from build123d import *

# Parameters (mm, degrees)
BOSS_EXTRUDE1_DEPTH = 3.175
SKETCH3_R           = 6.35
CUT_EXTRUDE2_DEPTH  = 4.175
CUT_EXTRUDE4_DEPTH  = 4.175
SKETCH4_W           = 6.35
SKETCH4_H           = 3.2258
CUT_EXTRUDE3_DEPTH  = 4.175


with BuildPart() as part:
    # Sketch1 → Boss-Extrude1 (new body)
    with BuildSketch(Plane(origin=(0, 0, 0), x_dir=(0, 0, -1), z_dir=(1, 0, 0))):
        with BuildLine():
            Line((20.308664328, 40.617328656), (43.157786531, 40.617328656))
            ThreePointArc((43.157786531, 40.617328656), (60.466141811, 27.624512399), (43.692194932, 13.948725661))
            Line((43.692194932, 13.948725661), (15.586038544, 7.228441393))
            Line((15.586038544, 7.228441393), (15.586038544, -35.582671344))
            Line((15.586038544, -35.582671344), (-17.791335672, -35.582671344))
            Line((-17.791335672, -35.582671344), (-17.791335672, 40.617328656))
            Line((-17.791335672, 40.617328656), (20.308664328, 40.617328656))
        make_face()
    extrude(amount=BOSS_EXTRUDE1_DEPTH)

    # Sketch3 → Cut-Extrude2 (cut, through all)
    with BuildSketch(Plane(origin=(3.175, 0, 0), x_dir=(0, 0, -1), z_dir=(1, 0, 0))):
        with Locations((50.788664328, 25.377328656)):
            Circle(SKETCH3_R)
    extrude(amount=-CUT_EXTRUDE2_DEPTH, mode=Mode.SUBTRACT)

    # Sketch5 → Cut-Extrude4 (cut, through all)
    with BuildSketch(Plane.ZY):
        Polygon((-15.586038544, 7.228441393), (-14.846971332, 2.578544694), (-14.846971332, -24.724280649), (-15.586038544, -32.273448946), align=None)
    extrude(amount=-CUT_EXTRUDE4_DEPTH, mode=Mode.SUBTRACT)

    # Sketch4 → Cut-Extrude3 (cut, through all)
    with BuildSketch(Plane(origin=(3.175, 0, 0), x_dir=(0, 0, -1), z_dir=(1, 0, 0))):
        with Locations((-10.627648564, -30.820171344)):
            Rectangle(SKETCH4_W, SKETCH4_H)
        with Locations((8.422351436, -30.820171344)):
            Rectangle(SKETCH4_W, SKETCH4_H)
    extrude(amount=-CUT_EXTRUDE3_DEPTH, mode=Mode.SUBTRACT)


solid = part.part
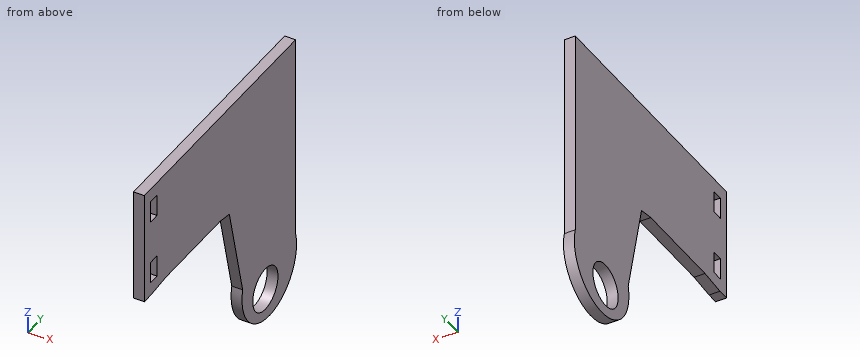
The listing builds one solid part. Answer for the finished solid, in the listing's coordinates (mm). Coordinates: 2 decimals unless noted, no trailing zeros. Order: outer loops, then holes, each group sorted by start corner. A loop starts at its lowest first (then second) coordinate and runs counter-clockwise, first axis right, second up.
Q1. Given P1, Ø1.6, axis at x = 1, y = -33.5, coming from the -Z side; P2, Ø1, axis at y = 25.5, z = -39, coming from the -X side; P3, Ø1.6, axis at x = 1, z = 10, coming from the +Y side, each flat-ended and moving along its own axis, determine where each tip first touches the part or whether it passes through.
Q2. A cutting plane is placed at B-B, the plane y = 21. Write down the section's boundary in (x, z) (1 decimal), and give its area (3 significant figures).
Q3. Consider line 1 (Y direction, x = 0.75, z = -11.5); line 2 (Y direction, x = 0.95, z = 14); line 3 (Z direction, x = 1.25, y = -18). Determine where each line is inside the solid, lowest interval first.
Q4. A cutting plane is placed at C-C, the plane x = 0.8. Write down the section's boundary in (y, z), and give its area (3 significant figures).
Q5. A cutting plane is placed at A-A, the plane z = 12. Write down the section's boundary in (x, y) (3 decimals), and give its area (3 significant figures).
Q6. A cutting plane is placed at D-D, the plane y = -19. Write down the section's boundary in (x, z) (3 decimals).
Answers follow:
1. P1: stops at z = -15.59
1. P2: stops at x = 0
1. P3: stops at y = 40.62
2. outline: (0, -58.9) - (3.2, -58.9) - (3.2, -55.4) - (0, -55.4) - close; (0, -46.2) - (3.2, -46.2) - (3.2, 17.8) - (0, 17.8) - close
2. area: 214 mm2
3. line 1: y = -35.58 to -32.43, -29.21 to 40.62
3. line 2: y = -35.58 to 40.62
3. line 3: z = -14.85 to 17.79
4. outline: (-35.58, -15.59) - (-32.27, -15.59) - (-24.72, -14.85) - (2.58, -14.85) - (7.23, -15.59) - (13.95, -43.69) arc R13.74 ccw (long way) to (40.62, -43.16) - (40.62, 17.79) - (-35.58, 17.79) - close; hole (-32.43, -11.6) - (-29.21, -11.6) - (-29.21, -5.25) - (-32.43, -5.25) - close; hole (-32.43, 7.45) - (-29.21, 7.45) - (-29.21, 13.8) - (-32.43, 13.8) - close; hole circle Ø12.7 at (25.38, -50.79)
4. area: 3,570 mm2
5. outline: (0, -35.583) - (3.175, -35.583) - (3.175, -32.433) - (0, -32.433) - close; (0, -29.207) - (3.175, -29.207) - (3.175, 40.617) - (0, 40.617) - close
5. area: 232 mm2
6. outline: (0, -14.847) - (3.175, -14.847) - (3.175, 17.791) - (0, 17.791) - close
